Check sheet for the modelled part. Datum: model origin and axes. Units: mm. A direction names the side the tool comes from. Round coordinates to 2 decimals unless told otherwise and drop trailing zeros. Write each loop counter-clockwise with the first axis right and the second up, starting at its lowest first coordinate (ties: lowest second). Pieces come first, ordered by that corner, then holes. Notation, with made-up numbers: M 46.5,70.25 L 89.5,70.25 A26 ccw 89.5,106.25 Z; hole C -2,37.5 d2. An arc over 180 degrees is marked long. Put each result on its own line as item: value.
```python
from build123d import *

# Parameters (mm, degrees)
PAD_DEPTH    = 20
POCKET_DEPTH = 232.483876


with BuildPart() as part:
    # Sketch → Pad (new body, symmetric)
    with BuildSketch(Plane.XY):
        with BuildLine():
            ThreePointArc((0, 25.5), (7.5, 33), (0, 40.5))
            Line((0, 40.5), (0, 50))
            ThreePointArc((17, 33), (12.020815, 45.020815), (0, 50))
            ThreePointArc((17, 33), (22.272078, 20.272078), (35, 15))
            Line((35, 15), (47.5, 15))
            Line((47.5, 15), (60, 15))
            ThreePointArc((65, 10), (63.535534, 13.535534), (60, 15))
            Line((65, 10), (65, 0))
            Line((65, 0), (0, 0))
            Line((0, 0), (0, 25.5))
        make_face()
    pad = extrude(amount=PAD_DEPTH, both=True)

    # Sketch001 → Pocket (cut, through all)
    with BuildSketch(Plane.XZ):
        with BuildLine():
            ThreePointArc((50, -5), (55, 0), (50, 5))
            Line((50, 5), (45, 5))
            ThreePointArc((45, 5), (40, 0), (45, -5))
            Line((45, -5), (50, -5))
        make_face()
    pocket = extrude(amount=-POCKET_DEPTH, mode=Mode.SUBTRACT)

    # Mirrored: Pad, Pocket across Sketch V_Axis
    add(pad.mirror(Plane(origin=(0, 0, 0), x_dir=(0, 0, 1), z_dir=(1, 0, 0))))
    add(pocket.mirror(Plane(origin=(0, 0, 0), x_dir=(0, 0, 1), z_dir=(1, 0, 0))), mode=Mode.SUBTRACT)


solid = part.part
```
1. Depth check by flat-ended pin: pin 1 Ø10 at (y, z) = (39.5, -16) entering from -X; pin 2 Ø3 at (y, z) = (39.5, 8) entering from -X; pin 3 Ø1.5 at (x, z) = (-3, 9.5) entering from +Y. Enter the tip coordinate at first touch or a pass-through.
Computed values:
pin 1: stops at x = -16.93
pin 2: stops at x = -16.25
pin 3: stops at y = 49.85
2. Cross-section at D-D (z = 12). Enter the section's corners in (x, y).
Computed values:
outline: M -65,0 L 65,0 L 65,10 A5 ccw 60,15 L 35,15 A18 cw 17,33 A17 ccw 0,50 A17 ccw -17,33 A18 cw -35,15 L -60,15 A5 ccw -65,10 Z; hole C 0,33 d15
3. Cross-section at A-A (z = 0). Enter the section's corners in (x, y), then the cut area to 3 significant figures.
Computed values:
outline: M -65,0 L -55,0 L -55,15 L -60,15 A5 ccw -65,10 Z; M -40,0 L 40,0 L 40,15 L 35,15 A18 cw 17,33 A17 ccw 0,50 A17 ccw -17,33 A18 cw -35,15 L -40,15 Z; M 55,0 L 65,0 L 65,10 A5 ccw 60,15 L 55,15 Z; hole C 0,33 d15
area: 2,520 mm2
4. Access from +Z, -Z, +X, -X, +Y, -Y to the whole of each face (thin tool, end or side, straight path). Record for faces 1 (the flat face through (-41.8, 15, -4.2)), 2 (the cylindrical face through (-40, 7, 0)), 3 (the flat face through (41.8, 15, -4.2)).
Computed values:
face 1: +Z, -Z, -X, +Y
face 2: +Y, -Y
face 3: +Z, -Z, +X, +Y
5. Scan lines: probe 1 along Z at (x, y) = (-49.5, 12); probe 2 along Y at (x, z) = (-45, -9); probe 3 along X at (y, z) = (28, 17.5). Record each from-to range of solid material in increasing order.
Computed values:
probe 1: z = -20 to -5, 5 to 20
probe 2: y = 0 to 15
probe 3: x = -17.71 to -5.59, 5.59 to 17.71
6. Cross-section at B-B (y = 7). Enter the section's corners in (x, z), then the cut area to 3 significant figures.
Computed values:
outline: M -65,-20 L 65,-20 L 65,20 L -65,20 Z; hole M -50,-5 L -45,-5 A5 ccw -45,5 L -50,5 A5 ccw Z; hole M 45,-5 L 50,-5 A5 ccw 50,5 L 45,5 A5 ccw Z
area: 4,940 mm2
7. Release check for a two-part mould opening along X. For faces 4 (the flat face through (-47, 7, -5)), 5 (the cylindrical face through (64, 13, 0)), 6 (the flat face through (-65, 5, 0)) record: +X half, -X half, draft (parallel to the pull), parting line (faces both ways), or undercut.
Computed values:
face 4: undercut
face 5: +X half
face 6: -X half
8. Cross-section at C-C (x = 53). Enter the section's corners in (y, z).
Computed values:
outline: M 0,-20 L 15,-20 L 15,-4 L 0,-4 Z; M 0,4 L 15,4 L 15,20 L 0,20 Z
